The model under review builds one solid part; all positions refer to its coordinate system, in mm. Face numbers are marked on the shaded views. A direction names the side the tool comes from. Coordinates: 2 decimals unless noted, no trailing zeros. Write each loop counter-clockwise with the first axis right and the second up, starting at its lowest first coordinate (ties: lowest second). Pieces come first, ordered by that corner, then holes. Notation, with made-up numbers: (35, 76.5) - (65, 76.5) arc R12 ccw to (65, 98.5) - close; hole circle Ø11 at (87.5, 49). An arc over 180 degrees is marked (long way). Return JSON: item names as keys, results as strings. Group by question number.
(1) We need section A-A on y = -10. State the section outline as (x, z) points, then the cut area to 3 significant figures.
(2) Draft analysis for pull direction X (two halves, no side actions). For the marked faces 1 and 2, state which applies: released by +X, released by -X, zero draft, split by the parting line, or undercut.
(3) We need section B-B on y = -18. State the section outline as (x, z) points, then the cut area to 3 significant figures.
(4) To check wall thickness, follow L1, parallel to X at y = -5, z = 0; L2, parallel to Z at x = -5.5, y = 7; L3, parallel to Z at x = 1.5, y = -21.5. State the ranges of each line that lie inside material, in increasing order. Write a range as from..to.
(5) Tool access review of the marked faces 3 and 4: name each direction out of +Z, -Z, +X, -X, +Y, -Y from which nothing blocks a thin tool from reaching the whole face with its end or side.
(6) For pin 1 Ø1.5 at (y, z) = (-25.5, 1) entering from +X; pin 2 Ø1 at (x, y) = (-6, -33.5) entering from +Z; pin 3 Ø6 at (x, y) = (-2, -33.5) entering from -Z, all flat-tipped, find the tip position at first contact; note any pin that passes through.
```python
from build123d import *

# Parameters (mm, degrees)
CHAMFER1_SIZE       = 4.28
CHAMFER1_SIZE2      = 4.038825392
SKETCH8_R           = 4.5
BOSS_EXTRUDE2_DEPTH = 9.5
FILLET2_R           = 3
SKETCH9_R           = 3
CUT_EXTRUDE2_DEPTH  = 66.346851097


with BuildPart() as part:
    # Sketch7 → Revolve1 (revolve)
    with BuildSketch(Plane(origin=(0, 0, 0), x_dir=(0, 0, -1), z_dir=(1, 0, 0))):
        Polygon((0, 0), (0, 22.597995894), (4.193169033, 22.597995894), (9.941146123, 0), align=None)
    revolve(axis=Axis((0, 0, 0), (0, 1, 0)))

    # Chamfer1
    chamfer1_edges = [part.edges().sort_by_distance(p)[0] for p in [
        (0, 0, 9.941146123),
    ]]
    chamfer1_side = [part.faces().sort_by_distance(p)[0] for p in [
        (0, 11.298997947, 7.067157578),
    ]]
    chamfer(chamfer1_edges, length=CHAMFER1_SIZE, length2=CHAMFER1_SIZE2, reference=chamfer1_side[0])

    # Sketch8 → Boss-Extrude2 (add)
    with BuildSketch(Plane.XZ):
        with Locations(Location((0, 0, 0), (0, 0, 270))):
            Circle(SKETCH8_R)
    extrude(amount=BOSS_EXTRUDE2_DEPTH)

    # Fillet2
    fillet2_edges = [part.edges().sort_by_distance(p)[0] for p in [
        (0, 4.147921891, 8.886089732),
    ]]
    fillet(fillet2_edges, radius=FILLET2_R)

    # Fillet3: read off the stored shape, not the designer's step
    # Fillet3 outline → Fillet3 (revolve)
    with BuildSketch(Plane.XY):
        with BuildLine():
            Line((4.5, 0), (4.5, -4.576097384))
            ThreePointArc((4.5, -4.576097384), (4.892931369, -2.076097384), (6.033834832, 0.182825888))
            Line((6.033834832, 0.182825888), (5.902320731, 0.182825888))
            Line((5.902320731, 0.182825888), (5.902320731, 0))
            Line((5.902320731, 0), (4.5, 0))
        make_face()
    revolve(axis=Axis((0, 0, 0), (0, 1, 0)))

    # Mirror3: part across plane


with BuildPart() as part_1:
    add(part.part)
    add(part.part.mirror(Plane(origin=(0, -9.5, 0), x_dir=(0, 0, 1), z_dir=(0, -1, 0))))

    # Sketch9 → Cut-Extrude2 (cut, through all)
    with BuildSketch(Plane(origin=(0, 22.597995894, 0), x_dir=(1, 0, 0), z_dir=(0, 1, 0))):
        with Locations(Location((0, 0, 0), (0, 0, 270))):
            Circle(SKETCH9_R)
    extrude(amount=-CUT_EXTRUDE2_DEPTH, mode=Mode.SUBTRACT)


solid = part_1.part
```
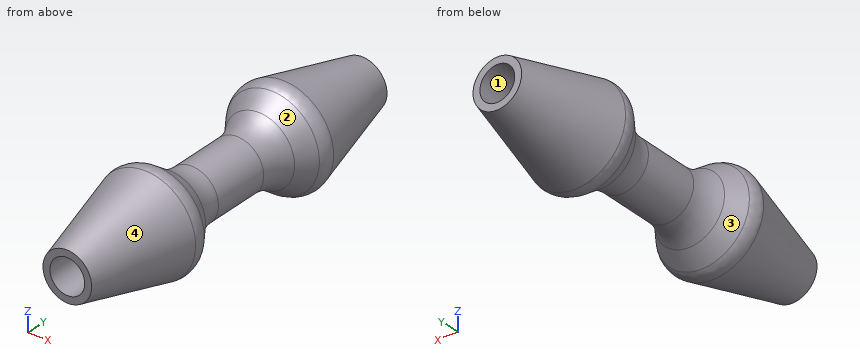
Ans:
{
 "1": {"outline": "circle Ø9 at (0, 0); hole circle Ø6 at (0, 0)", "area": "35.3 mm²"},
 "2": {"face 1": "undercut", "face 2": "split by the parting line"},
 "3": {"outline": "circle Ø10.65 at (0, 0); hole circle Ø6 at (0, 0)", "area": "60.9 mm²"},
 "4": {"L1": "-4.5..-3, 3..4.5", "L2": "-6.03..6.03", "L3": "-7.55..-2.6, 2.6..7.55"},
 "5": {"face 3": "none", "face 4": "-Y"},
 "6": {"pin 1": "x = 8.43", "pin 2": "z = 3.01", "pin 3": "z = -6.91"}
}
